from build123d import *

# Parameters (mm, degrees)
SKETCH1_R           = 25.4
SKETCH1_R_2         = 4.05
BOSS_EXTRUDE1_DEPTH = 1.1
SKETCH2_R           = 0.69375
BOSS_EXTRUDE2_DEPTH = 1.5875
BOSS_EXTRUDE3_START = 0.5
SKETCH3_R           = 25.4
SKETCH3_R_2         = 3.9
BOSS_EXTRUDE3_DEPTH = 0.5


with BuildPart() as part:
    # Sketch1 → Boss-Extrude1 (new body)
    with BuildSketch(Plane.XY):
        Circle(SKETCH1_R)
        with Locations((0, 20.35)):
            Circle(SKETCH1_R_2, mode=Mode.SUBTRACT)
        with Locations((14.389622997, 14.389622997)):
            Circle(SKETCH1_R_2, mode=Mode.SUBTRACT)
        with Locations((20.35, 0)):
            Circle(SKETCH1_R_2, mode=Mode.SUBTRACT)
        with Locations((14.389622997, -14.389622997)):
            Circle(SKETCH1_R_2, mode=Mode.SUBTRACT)
        with Locations((0, -20.35)):
            Circle(SKETCH1_R_2, mode=Mode.SUBTRACT)
        with Locations((-14.389622997, -14.389622997)):
            Circle(SKETCH1_R_2, mode=Mode.SUBTRACT)
        with Locations((-20.35, 0)):
            Circle(SKETCH1_R_2, mode=Mode.SUBTRACT)
        with Locations((-14.389622997, 14.389622997)):
            Circle(SKETCH1_R_2, mode=Mode.SUBTRACT)
    extrude(amount=BOSS_EXTRUDE1_DEPTH)

    # Sketch2 → Boss-Extrude2 (add)
    with BuildSketch(Plane.XY.offset(1.1)):
        Circle(SKETCH2_R)
    extrude(amount=BOSS_EXTRUDE2_DEPTH)

    # Sketch3 → Boss-Extrude3 (add)
    with BuildSketch(Plane(origin=(0, 0, 0), x_dir=(-1, 0, 0), z_dir=(0, 0, -1)).offset(BOSS_EXTRUDE3_START)):
        Circle(SKETCH3_R)
        with Locations((0, 20.35)):
            Circle(SKETCH3_R_2, mode=Mode.SUBTRACT)
        with Locations((14.389622997, 14.389622997)):
            Circle(SKETCH3_R_2, mode=Mode.SUBTRACT)
        with Locations((20.35, 0)):
            Circle(SKETCH3_R_2, mode=Mode.SUBTRACT)
        with Locations((14.389622997, -14.389622997)):
            Circle(SKETCH3_R_2, mode=Mode.SUBTRACT)
        with Locations((0, -20.35)):
            Circle(SKETCH3_R_2, mode=Mode.SUBTRACT)
        with Locations((-14.389622997, -14.389622997)):
            Circle(SKETCH3_R_2, mode=Mode.SUBTRACT)
        with Locations((-20.35, 0)):
            Circle(SKETCH3_R_2, mode=Mode.SUBTRACT)
        with Locations((-14.389622997, 14.389622997)):
            Circle(SKETCH3_R_2, mode=Mode.SUBTRACT)
    extrude(amount=-BOSS_EXTRUDE3_DEPTH)


solid = part.part
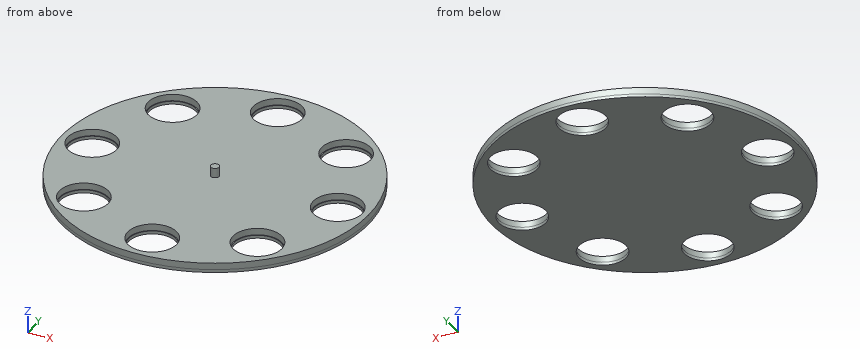
The listing builds one solid part. Answer for the finished solid, in the listing's coordinates (mm). Coordinates: 2 decimals unless noted, no trailing zeros. Write each loop counter-clockwise with the first axis right and the second up, starting at its lowest first coordinate (ties: lowest second). Pieces come first, ordered by that corner, then holes. Notation, with made-up numbers: M -6,70 L 53,70 A8 ccw 53,78 Z; hole C 49,8 d9. An arc over 180 degrees is marked long. Write each question's results on one line, items separated by ' | '.
Item 1: Given P1, Ø15, axis at x = -2, y = 10.5, coming from the +Z side; P2, Ø7, axis at x = 0, y = -20.35, coming from the +Z side; P3, Ø1, axis at y = 16, z = 1, coming from the +X side; P4, Ø1.5, axis at y = 11, z = 1, coming from the +X side, each flat-ended and moving along its own axis, determine where each tip first touches the part or whether it passes through.
Answer below:
P1: z = 1.1 | P2: through | P3: x = 20.12 | P4: x = 23.24
Item 2: The part is cut by section D-D on z = 2.2. Determine the outline of the cut face in (x, y), and give its area (3 significant figures).
Answer below:
outline: C 0,0 d1.39 | area: 1.51 mm2
Item 3: The part is cut by section B-B on x = -20.35. Determine the outline of the cut face in (y, z), and give its area (3 significant figures).
Answer below:
outline: M -15.2,-0.5 L -3.9,-0.5 L -3.9,0 L -4.05,0 L -4.05,1.1 L -15.2,1.1 Z; M 3.9,-0.5 L 15.2,-0.5 L 15.2,1.1 L 4.05,1.1 L 4.05,0 L 3.9,0 Z | area: 35.8 mm2
Item 4: Consider probe 1 along X at (y, z) = (-12, -0.1); probe 2 along Z at (x, y) = (-12, 22); probe 3 along Y at (x, z) = (22.5, 0.55). Determine where each line is inside the solid, lowest interval first. Write a range as [from, to].
Answer below:
probe 1: [-22.39, -17.47], [-11.31, 11.31], [17.47, 22.39] | probe 2: [-0.5, 1.1] | probe 3: [-11.79, -3.43], [3.43, 11.79]
Item 5: The part is cut by section A-A on y = 0. Determine the outline of the cut face in (x, z).
Answer below:
outline: M -25.4,-0.5 L -24.25,-0.5 L -24.25,0 L -24.4,0 L -24.4,1.1 L -25.4,1.1 Z; M -16.45,-0.5 L 16.45,-0.5 L 16.45,0 L 16.3,0 L 16.3,1.1 L 0.69,1.1 L 0.69,2.69 L -0.69,2.69 L -0.69,1.1 L -16.3,1.1 L -16.3,0 L -16.45,0 Z; M 24.25,-0.5 L 25.4,-0.5 L 25.4,1.1 L 24.4,1.1 L 24.4,0 L 24.25,0 Z
